Design review of the part built by this model. Coordinates are the model's own, in mm. A direction names the side the tool comes from. Coordinates: 2 decimals unless noted, no trailing zeros. Order: outer loops, then holes, each group sorted by start corner. A loop starts at its lowest first (then second) coordinate and runs counter-clockwise, first axis right, second up. Notation, with made-up numbers: (-27.75, 63) - (-0.75, 63) arc R19 ccw to (-0.75, 83) - close; hole circle Ø6 at (89.5, -11). An arc over 180 degrees is marked (long way). Write each question's results on one line, items separated by ' | '. Start each with the question number.
Solid Edge part; units mm, degrees
sketch "Sketch1" plane through (0, 0, 0) normal (0, -1, 0) x (1, 0, 0)
  line L0 (350, 0) -> (350, 350)
  line L1 (350, 350) -> (0, 350)
  line L2 (0, 350) -> (0, 0)
  line L3 (0, 0) -> (350, 0)
extrude "Protrusion1" add sketch "Sketch1" against normal blind 20
sketch "Sketch2" plane through (250, 0, 250) normal (0, -1, 0) x (0, 0, 1)
  line L0 (-175, 250) -> (-175, 230)
  line L1 (-175, 230) -> (25, 230)
  line L2 (25, 230) -> (25, 250)
  line L3 (25, 250) -> (-175, 250)
  dimension "D1" = 175
  dimension "D2" = 175
extrude "Extrusionsausschnitt_1" cut sketch "Sketch2" against normal blind 67.8542
hole "Bohrung_1" at (185, 0, 205) direction (0, 1, 0) diameter 10.5 end up to next start chamfer 1 start chamfer angle 45
hole "Hole1" at (185, 0, 145) direction (0, 1, 0) diameter 10.5 end up to next start chamfer 1 start chamfer angle 45
(1) Take a section at A-A (x = 185). State the section outline as (y, z) points.
(2) Mouldability with a two-part tool opening along Z and no side actions: class faces 3 (the face through (177, 10, 350)), 4 (the face through (186.6, 10.4, 140)), 5 (the face through (10, 10, 275)), 6 (the face through (173, 10, 0)) as +Z half, -Z half, draft (parallel to the pull), parting line (faces both ways), or undercut.
(3) Tool access review of faces 1 (the face through (186.6, 10.4, 200)), 2 (the face through (10, 10, 75)): name each direction out of +Z, -Z, +X, -X, +Y, -Y from which nothing blocks a thin tool from reaching the whole face with its end or side.
(4) Take a section at C-C (y = 4.25). State the section outline as (x, z) points.
(5) Clearance check with flat-ended pins moving along their axes: pin 1 (12 mm diameter, centred on x = 185, z = 205, fed in from -Y); pin 2 (10 mm diameter, centred on y = 7, z = 137, fed in from -X). State where each tip first meets the part, or that it passes through.
(6) Take a section at B-B (z = 145). State the section outline as (x, y) points, plus the area to 3 significant figures.
(7) To check wall thickness, follow line 1 along Z through (x, y) = (185, 12); line 2 along X through (y, z) = (12.75, 205); line 3 along X through (y, z) = (8.5, 215.5). State the ranges of each line that lie inside material, in increasing order. Write a range as [from, to].
Worked out:
1) outline: (0, 0) - (20, 0) - (20, 139.75) - (1, 139.75) - (0, 138.75) - close; (0, 151.25) - (1, 150.25) - (20, 150.25) - (20, 199.75) - (1, 199.75) - (0, 198.75) - close; (0, 211.25) - (1, 210.25) - (20, 210.25) - (20, 350) - (0, 350) - close
2) face 3: +Z half | face 4: undercut | face 5: undercut | face 6: -Z half
3) face 1: +Y, -Y | face 2: -X, +Y, -Y
4) outline: (0, 0) - (350, 0) - (350, 350) - (0, 350) - (0, 275) - (20, 275) - (20, 75) - (0, 75) - close; hole circle Ø10.5 at (185, 145); hole circle Ø10.5 at (185, 205)
5) pin 1: y = 0.25 | pin 2: x = 20
6) outline: (20, 0) - (178.75, 0) - (179.75, 1) - (179.75, 20) - (20, 20) - close; (190.25, 1) - (191.25, 0) - (350, 0) - (350, 20) - (190.25, 20) - close | area: 6,390 mm^2
7) line 1: [0, 139.75], [150.25, 199.75], [210.25, 350] | line 2: [20, 179.75], [190.25, 350] | line 3: [20, 350]
